Read the model definition and answer for the solid it produces. Units are mm, in the model's axes. A direction names the side the tool comes from. Coordinates: 2 decimals unless noted, no trailing zeros. Use one line per item in the form item = value. Start each with the question number.
1. The part is cut by section A-A (z = 2.7). Give the number of separate pieces and of enclosed holes in the cut face, plus the area to 3 significant figures.
2. Find the intervals of material crossed by probe 1 along Y at (x, z) = (-175, 1.9); probe 2 along Y at (x, z) = (174.5, 2.9); probe 3 along Y at (x, z) = (-96, 2.2), in increasing order. Write a range as [from, to].
3. For a pull along X with two mould halves and no side action, classify faces 1 (the flat face through (1, 1, 4)), 2 (the cylindrical face through (-14.612, -14.918, 2.028)), 3 (the flat face through (-51.071, -12.317, 2.028)) as released by +X, released by -X, zero draft, split by the parting line, or undercut.
4. A flat-ended cylindrical pin translates along its axis: pin 1 (2 mm diameter, centred on y = 17.5, z = 3.5, fed in from -X). Find the tip coordinate at first contact, or state that the pin passes through.
5. A tool of negligible diameter and unlimited length cuts with its end or side. For faces 4 (the cylindrical face through (185.414, 27.066, 1.972)), 5 (the cylindrical face through (140.125, -22.247, 2.028)), 6 (the flat face through (-29.153, 29.125, 1.972)), from which of +Z, -Z, +X, -X, +Y, -Y can it reach the whole face along a straight path? Write none if from no direction.
from build123d import *

# Parameters (mm, degrees)
SKETCH1_R              = 11.1125
SKETCH1_R_2            = 15
SKETCH1_R_3            = 1.6
BOSS_EXTRUDE1_DEPTH    = 4
M3_5_CLEARANCE_HOLE1_D = 3.9
CUT_EXTRUDE1_DEPTH     = 10
BOSS_EXTRUDE2_START    = -4
BOSS_EXTRUDE2_DEPTH    = 4
FILLET1_R              = 2
FILLET2_R              = 80


with BuildPart() as part:
    # Sketch1 → Boss-Extrude1 (new body)
    with BuildSketch(Plane.XY):
        with BuildLine():
            Line((-172.834121622, 37.437400696), (175.998333346, 17.256280804))
            ThreePointArc((175.998333346, 17.256280804), (192.285135135, 0), (175.998333346, -17.256280804))
            Line((175.998333346, -17.256280804), (-172.834121622, -37.437400696))
            ThreePointArc((-172.834121622, -37.437400696), (-212.5, 0), (-172.834121622, 37.437400696))
        make_face()
        with Locations((175, 0)):
            Circle(SKETCH1_R, mode=Mode.SUBTRACT)
        with Locations((-175, 0)):
            Circle(SKETCH1_R_2, mode=Mode.SUBTRACT)
        with Locations((-132.5, 30.095576829)):
            Circle(SKETCH1_R_3, mode=Mode.SUBTRACT)
        with Locations((-67.805059302, 26.352758935)):
            Circle(SKETCH1_R_3, mode=Mode.SUBTRACT)
        with Locations((-3.110118604, 22.60994104)):
            Circle(SKETCH1_R_3, mode=Mode.SUBTRACT)
        with Locations((61.584822094, 18.867123146)):
            Circle(SKETCH1_R_3, mode=Mode.SUBTRACT)
        with Locations((126.279762792, 15.124305251)):
            Circle(SKETCH1_R_3, mode=Mode.SUBTRACT)
        with Locations(Location((126.279762792, -15.124305251, 0), (0, 0, 180))):
            Circle(SKETCH1_R_3, mode=Mode.SUBTRACT)
        with Locations(Location((61.584822094, -18.867123146, 0), (0, 0, 180))):
            Circle(SKETCH1_R_3, mode=Mode.SUBTRACT)
        with Locations(Location((-3.110118604, -22.60994104, 0), (0, 0, 180))):
            Circle(SKETCH1_R_3, mode=Mode.SUBTRACT)
        with Locations(Location((-67.805059302, -26.352758935, 0), (0, 0, 180))):
            Circle(SKETCH1_R_3, mode=Mode.SUBTRACT)
        with Locations(Location((-132.5, -30.095576829, 0), (0, 0, 180))):
            Circle(SKETCH1_R_3, mode=Mode.SUBTRACT)
    extrude(amount=BOSS_EXTRUDE1_DEPTH)

    # M3.5 Clearance Hole1 (through all)
    with Locations(Plane.XY.offset(4)):
        with Locations((-197.5, 0), (-175, 22.5), (-152.5, 0), (-175, -22.5)):
            Hole(M3_5_CLEARANCE_HOLE1_D / 2)

    # Sketch7 → Cut-Extrude1 (cut)
    with BuildSketch(Plane.XY.offset(4)):
        with BuildLine():
            Line((15.991284585, 5.612221232), (28.312344657, -2.287027054))
            ThreePointArc((28.312344657, -2.287027054), (31.73354052, -11.048707916), (24.456630921, -17.008424298))
            Line((24.456630921, -17.008424298), (12.632145333, -17.692510191))
            ThreePointArc((12.632145333, -17.692510191), (6.849401654, -15.679997443), (4.183445797, -10.167918763))
            Line((4.183445797, -10.167918763), (3.686871313, -1.584584585))
            ThreePointArc((3.686871313, -1.584584585), (7.634498428, 5.782998459), (15.991284585, 5.612221232))
        make_face()
        with BuildLine():
            Line((-11.941116444, -8.477289375), (-12.966479952, 9.246210209))
            ThreePointArc((-12.966479952, 9.246210209), (-15.914080917, 14.997692214), (-22.150280177, 16.694075277))
            Line((-22.150280177, 16.694075277), (-80.189531309, 7.909919122))
            ThreePointArc((-80.189531309, 7.909919122), (-86.992376567, 0), (-80.189531309, -7.909919122))
            Line((-80.189531309, -7.909919122), (-21.124916668, -16.849262551))
            ThreePointArc((-21.124916668, -16.849262551), (-14.538255469, -14.851468272), (-11.941116444, -8.477289375))
        make_face()
        with BuildLine():
            Line((-7.35411028, -2.925540775), (-8.509245415, 17.04107293))
            ThreePointArc((-8.509245415, 17.04107293), (-5.593466237, 20.314944), (-2.319595167, 17.399164822))
            Line((-2.319595167, 17.399164822), (-1.164460032, -2.567448883))
            ThreePointArc((-1.164460032, -2.567448883), (-4.08023921, -5.841319953), (-7.35411028, -2.925540775))
        make_face()
    extrude(amount=-CUT_EXTRUDE1_DEPTH, mode=Mode.SUBTRACT)

    # Sketch9 → Boss-Extrude2 (add)
    with BuildSketch(Plane.XY.offset(4).offset(BOSS_EXTRUDE2_START)):
        with BuildLine():
            Line((192.169038897, 2), (203.930952283, 2))
            ThreePointArc((203.930952283, 2), (183.947829075, 27.585074857), (152.751498531, 18.60118766))
            Line((152.751498531, 18.60118766), (147.934334346, 18.87987666))
            ThreePointArc((147.934334346, 18.87987666), (208, 0), (147.934334346, -18.87987666))
            Line((147.934334346, -18.87987666), (152.751498531, -18.60118766))
            ThreePointArc((152.751498531, -18.60118766), (183.947829075, -27.585074857), (203.930952283, -2))
            Line((203.930952283, -2), (192.169038897, -2))
            ThreePointArc((192.169038897, -2), (192.285135135, 0), (192.169038897, 2))
        make_face()
    extrude(amount=BOSS_EXTRUDE2_DEPTH)

    # Fillet1
    fillet1_edges = [part.edges().sort_by_distance(p)[0] for p in [
        (192.169038897, 2, 2),
        (192.169038897, -2, 2),
        (203.930952283, -2, 2),
        (152.751498531, -18.60118766, 2),
        (152.751498531, 18.60118766, 2),
        (203.930952283, 2, 2),
    ]]
    fillet(fillet1_edges, radius=FILLET1_R)

    # Fillet2
    fillet2_edges = [part.edges().sort_by_distance(p)[0] for p in [
        (147.934334346, -18.87987666, 2),
        (147.934334346, 18.87987666, 2),
    ]]
    fillet(fillet2_edges, radius=FILLET2_R)


solid = part.part
Computed values:
q1.separate_pieces = 1
q1.enclosed_holes = 21
q1.area = 19,000 mm²
q2.probe_1 = [-37.5, -24.45], [-20.55, -15], [15, 20.55], [24.45, 37.5]
q2.probe_2 = [-33, -29], [-17.34, -11.1], [11.1, 17.34], [29, 33]
q2.probe_3 = [-32.99, 32.99]
q3.face_1 = zero draft
q3.face_2 = undercut
q3.face_3 = undercut
q4.pin_1 = -208.67
q5.face_4 = +Z, -Z
q5.face_5 = +Z, -Z, -Y
q5.face_6 = +Z, -Z, +Y
